```python
from build123d import *

# Parameters (mm, degrees)
BOSS_EXTRUDE1_DEPTH = 10
SKETCH2_R           = 2.5
SKETCH2_R_2         = 32.5
CUT_EXTRUDE1_DEPTH  = 11
SKETCH3_R           = 3.25
CUT_EXTRUDE2_DEPTH  = 11


with BuildPart() as part:
    # Sketch1 → Boss-Extrude1 (new body)
    with BuildSketch(Plane(origin=(0, 0, 0), x_dir=(1, 0, 0), z_dir=(0, 1, 0))):
        with BuildLine():
            Line((100, 45), (-55, 45))
            ThreePointArc((-55, 45), (-100, 0), (-55, -45))
            Line((-55, -45), (100, -45))
            Line((100, -45), (100, 45))
        make_face()
    extrude(amount=BOSS_EXTRUDE1_DEPTH)

    # Sketch2 → Cut-Extrude1 (cut, through all)
    with BuildSketch(Plane(origin=(0, 10, 0), x_dir=(1, 0, 0), z_dir=(0, 1, 0))):
        with Locations((-92.5, 0)):
            Circle(SKETCH2_R)
        with Locations((-87.475952642, 18.75)):
            Circle(SKETCH2_R)
        with Locations((-73.75, 32.475952642)):
            Circle(SKETCH2_R)
        with Locations((-55, 0)):
            Circle(SKETCH2_R_2)
        with Locations((-55, 37.5)):
            Circle(SKETCH2_R)
        with Locations((-36.25, 32.475952642)):
            Circle(SKETCH2_R)
        with Locations((-22.524047358, 18.75)):
            Circle(SKETCH2_R)
        with Locations((-17.5, 0)):
            Circle(SKETCH2_R)
        with Locations((-22.524047358, -18.75)):
            Circle(SKETCH2_R)
        with Locations((-36.25, -32.475952642)):
            Circle(SKETCH2_R)
        with Locations((-55, -37.5)):
            Circle(SKETCH2_R)
        with Locations((-73.75, -32.475952642)):
            Circle(SKETCH2_R)
        with Locations((-87.475952642, -18.75)):
            Circle(SKETCH2_R)
    extrude(amount=-CUT_EXTRUDE1_DEPTH, mode=Mode.SUBTRACT)

    # Sketch3 → Cut-Extrude2 (cut, through all)
    with BuildSketch(Plane(origin=(0, 10, 0), x_dir=(1, 0, 0), z_dir=(0, 1, 0))):
        with Locations((80, 15)):
            Circle(SKETCH3_R)
        with Locations((50, 15)):
            Circle(SKETCH3_R)
        with Locations((50, -15)):
            Circle(SKETCH3_R)
        with Locations((80, -15)):
            Circle(SKETCH3_R)
    extrude(amount=-CUT_EXTRUDE2_DEPTH, mode=Mode.SUBTRACT)


solid = part.part
```
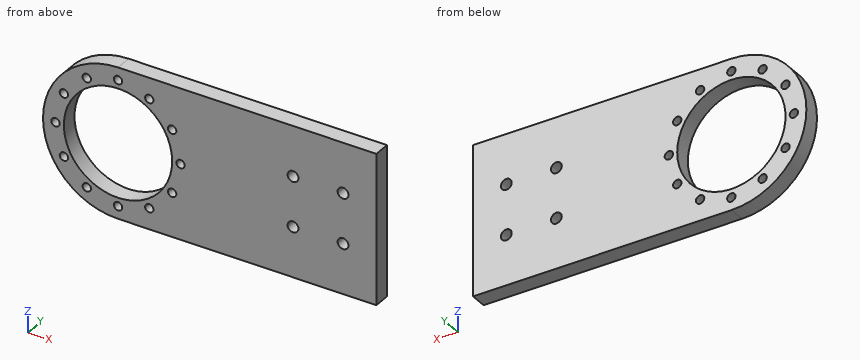
The listing builds one solid part. Answer for the finished solid, in the listing's coordinates (mm). Coordinates: 2 decimals unless noted, no trailing zeros. Loops run counter-clockwise (first coordinate to the right, second up) from the corner with the lowest first, then second, coordinate; pieces in that order, holes last. Notation, with made-up numbers: M 76.25,42 L 119.25,42 A23 ccw 119.25,53 Z; hole C -1,-23 d6. An arc over 180 degrees is marked long. Answer as CSV lines item,"result". Start each with the question number.
(1) The part is cut by section B-B (x = -73.75). Give the vertices of the cut face in (y, z).
(2) The part is cut by section C-C (z = -37.5). Give the vertices of the cut face in (x, y), and give its area (3 significant figures).
(3) The part is cut by section D-D (y = 6.5). State how many separate pieces and enclosed holes the cut face has, and give its area (3 significant figures).
(4) Find the intervals of material crossed by L1, parallel to Z at x = 50, y = 6.5; L2, parallel to X at y = 9, z = -13; L3, parallel to Z at x = 49, y = 3.5, in increasing order. Write a range as [from, to].
(5) The part is cut by section A-A (x = 80). Give the vertices of the cut face in (y, z).
(6) Given pin 1 (8 mm diameter, centred on x = -87.48, z = -18.75, fed in from +Y); pin 2 (4 mm diameter, centred on y = 7.5, z = -21, fed in from -X); pin 3 (5 mm diameter, centred on y = 8.5, z = -27.5, fed in from -X), each flat-ended and moving along its own axis, determine where each tip first touches the part or whether it passes through.
Determined:
1,outline,"M 0,-40.91 L 10,-40.91 L 10,-34.98 L 0,-34.98 Z; M 0,-29.98 L 10,-29.98 L 10,-26.55 L 0,-26.55 Z; M 0,26.55 L 10,26.55 L 10,29.98 L 0,29.98 Z; M 0,34.98 L 10,34.98 L 10,40.91 L 0,40.91 Z"
2,outline,"M -79.87,0 L -57.5,0 L -57.5,10 L -79.87,10 Z; M -52.5,0 L 100,0 L 100,10 L -52.5,10 Z"
2,area,"1,750 mm2"
3,separate pieces,"1"
3,enclosed holes,"17"
3,area,"13,400 mm2"
4,L1,"[-45, -18.25], [-11.75, 11.75], [18.25, 45]"
4,L2,"[-98.08, -84.79], [-25.21, 47.44], [52.56, 77.44], [82.56, 100]"
4,L3,"[-45, -18.09], [-11.91, 11.91], [18.09, 45]"
5,outline,"M 0,-45 L 10,-45 L 10,-18.25 L 0,-18.25 Z; M 0,-11.75 L 10,-11.75 L 10,11.75 L 0,11.75 Z; M 0,18.25 L 10,18.25 L 10,45 L 0,45 Z"
6,pin 1,"y = 10"
6,pin 2,"x = -95.79"
6,pin 3,"x = -92.42"
